The figure shows three views and two pictorial views of one solid part (mm, origin at its lowest corner). Answer the questions. Round coordinates to 2 decimals unless told otherwise and drop trailing zeros. Order: outer loops, then holes, each group sorted by start corner. A loop starts at its lowest first (then second) coordinate and runs counter-clockwise, first axis right, second up.
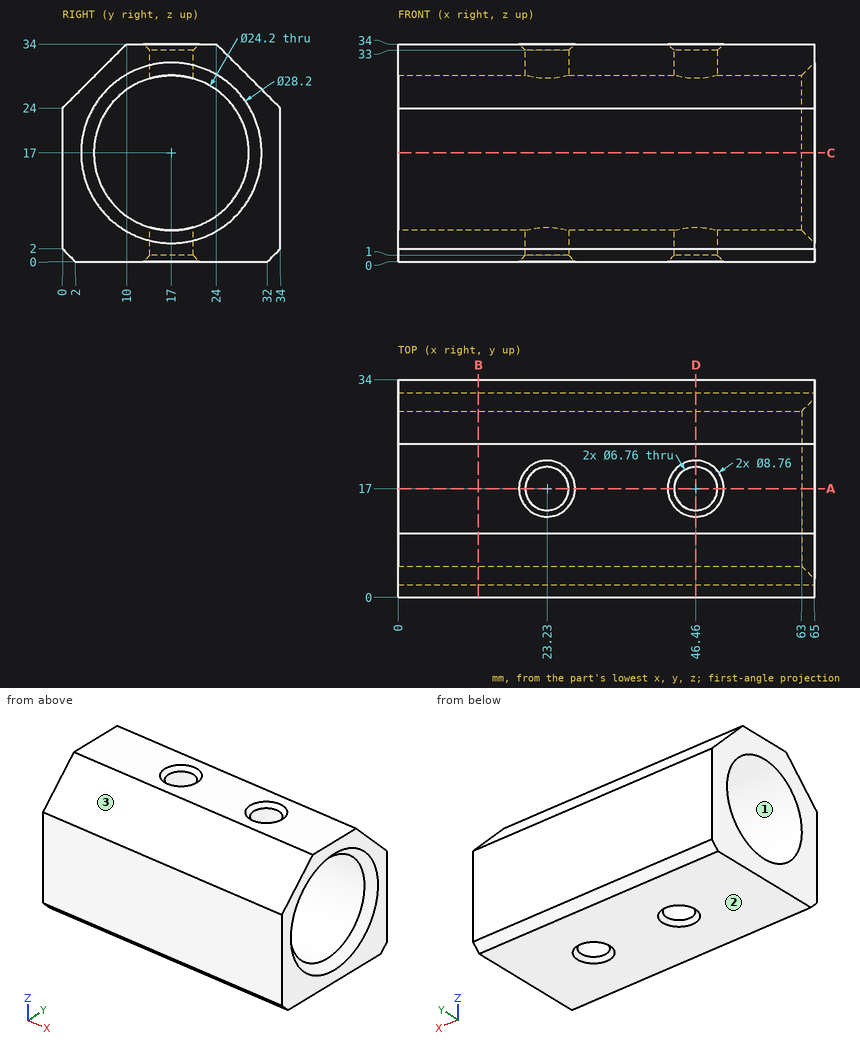
Item 1: Find section D-D (x = 46.46). Write down the section's boundary in (y, z), plus the area to 3 significant figures.
Item 2: Find the intervals of material crossed by line 1 along X through (y, z) = (17, 2.55); line 2 along Y through (x, z) = (31, 17); line 3 along X through (y, z) = (17, 3), in increasing order.
Item 3: Find section C-C (z = 17). Write down the section's boundary in (x, y), plus the area to 3 significant figures.
Item 4: Given pin 1 (6 mm diameter, centred on y = 18, z = 4, fed in from +X); pin 2 (1 mm diameter, centred on x = 17, z = 28.5, fed in from -Y), each flat-ended and moving along its own axis, determine where each tip first touches the part or whether it passes through.
Item 5: Find section A-A (y = 17). State how many separate pieces and enclosed holes the cut face has, plus the area to 3 significant figures.
Item 6: For a pull along Z with two mould halves and no side action, classify the marked faces 1, 2 and 3 as released by +Z, released by -Z, zero draft, split by the parting line, or undercut.
Item 7: Find section B-B (x = 12.5). Write down the section's boundary in (y, z).
Model answer:
1. outline: (0, 2) - (2, 0) - (12.62, 0) - (13.62, 1) - (13.62, 5.38) arc R12.1 cw to (13.62, 28.62) - (13.62, 33) - (12.62, 34) - (10, 34) - (0, 24) - close; (20.38, 1) - (21.38, 0) - (32, 0) - (34, 2) - (34, 24) - (24, 34) - (21.38, 34) - (20.38, 33) - (20.38, 28.62) arc R12.1 cw to (20.38, 5.38) - close
1. area: 522 mm2
2. line 1: x = 0 to 19.85, 26.61 to 43.08, 49.84 to 65
2. line 2: y = 0 to 4.9, 29.1 to 34
2. line 3: x = 0 to 19.85, 26.61 to 43.08, 49.84 to 64.9
3. outline: (0, 0) - (65, 0) - (65, 2.9) - (63, 4.9) - (0, 4.9) - close; (0, 29.1) - (63, 29.1) - (65, 31.1) - (65, 34) - (0, 34) - close
3. area: 633 mm2
4. pin 1: stops at x = 65
4. pin 2: stops at y = 4
5. separate pieces: 6
5. enclosed holes: 0
5. area: 497 mm2
6. face 1: undercut
6. face 2: released by -Z
6. face 3: released by +Z
7. outline: (0, 2) - (2, 0) - (32, 0) - (34, 2) - (34, 24) - (24, 34) - (10, 34) - (0, 24) - close; hole circle Ø24.2 at (17, 17)
